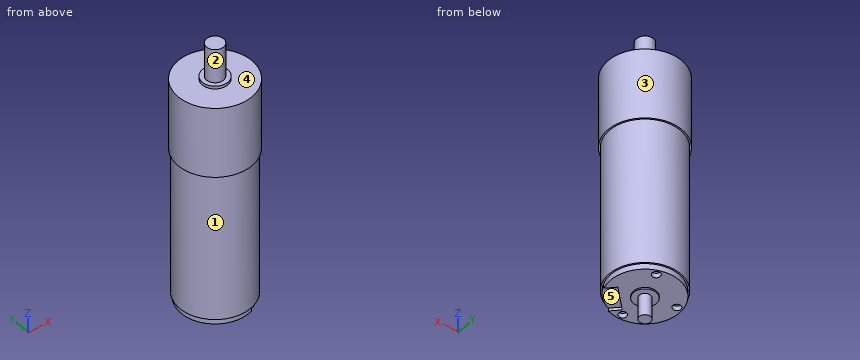
from build123d import *

# Parameters (mm, degrees)
SKETCH3_R          = 2.8
CUT_EXTRUDE2_DEPTH = 3.25
CUT_EXTRUDE3_DEPTH = 2


with BuildPart() as part:
    # Sketch1 → Revolve1 (revolve)
    with BuildSketch(Plane(origin=(0, 0, 0), x_dir=(0, 0, -1), z_dir=(1, 0, 0)), mode=Mode.PRIVATE) as revolve1_sk:
        Polygon((-76, 0), (124.5, 0), (124.5, 4), (109, 4), (109, 8), (108, 8), (108, 24), (104, 24), (104, 25), (0, 25), (0, 26), (-50, 26), (-50, 9), (-52, 9), (-52, 6), (-76, 6), align=None)
    revolve(revolve1_sk.sketch.rotate(Axis((0, 0, 76), (0, 0, -1)), 180), axis=Axis((0, 0, 76), (0, 0, -1)))

    # Sketch3 → Cut-Extrude2 (cut)
    with BuildSketch(Plane.XY.offset(-108)):
        with Locations(Location((6.767859423, 19.032500593, 0), (0, 0, 180))):
            Circle(SKETCH3_R)
        with Locations(Location((-19.905985431, 3.433910891, 0), (0, 0, 180))):
            Circle(SKETCH3_R)
        with Locations(Location((0, -20.2, 0), (0, 0, 180))):
            Circle(SKETCH3_R)
    extrude(amount=CUT_EXTRUDE2_DEPTH, mode=Mode.SUBTRACT)

    # Sketch4 → Cut-Extrude3 (cut)
    with BuildSketch(Plane(origin=(0, 0, -108), x_dir=(-1, 0, 0), z_dir=(0, 0, -1))):
        Polygon((-22.506441861, -8.334271099), (-16.973308635, -2.811902197), (-2.844949371, -16.967800773), (-8.378082597, -22.490169675), (-11.338488517, -25.444816332), (-25.466847781, -11.288917756), align=None)
    extrude(amount=-CUT_EXTRUDE3_DEPTH, mode=Mode.SUBTRACT)


solid = part.part
Could you check a few things on this model? Use its own coordinates, in mm. Face numbers are marked on the shaded views. A direction names the side the tool comes from. Give positions to 0.01 mm unless a question says otherwise; leave off trailing zeros. Loops run counter-clockwise (first coordinate to the right, second up) from the corner with the lowest first, then second, coordinate; pieces in that order, holes last. Notation, with made-up numbers: M -35.5,-1 L -9.5,-1 A12 ccw -9.5,8 Z; hole C -34,-11 d6. An arc over 180 degrees is marked long. Answer as a JSON object with one key per item and string values.
Q1. Suppose I cut it at C-C, the plane y = -20.2. List the corners of the cut face in (x, z) for me.
Values found:
{"outline": "M -16.37,0 L -14.73,0 L -14.73,-104 L -12.96,-104 L -12.96,-108 L -2.8,-108 L -2.8,-104.75 L 2.8,-104.75 L 2.8,-108 L 6.08,-108 L 6.08,-106 L 12.96,-106 L 12.96,-104 L 14.73,-104 L 14.73,0 L 16.37,0 L 16.37,50 L -16.37,50 Z"}
Q2. For P1, Ø15.5, axis at x = 11, y = -13.5, coming from the -Z side; P2, Ø6.5, axis at x = 6.77, y = 19.03, coming from the +Z side; P3, Ø3, axis at y = -14, z = -33.5, coming from the +X side, each with a flat end and sliding along its axis, tell me the tip position at first contact or that it passes through.
Values found:
{"P1": "stops at z = -108", "P2": "stops at z = 50", "P3": "stops at x = 21.65"}
Q3. If we mould it in two halves opening along X, with no side actions, what happens to the marked faces 3, 4 and 5? For each: pulls with the +X half, pulls with the -X half, needs draft (parallel to the pull), parting line crosses it, or undercut.
Values found:
{"face 3": "parting line crosses it", "face 4": "needs draft", "face 5": "undercut"}
Q4. If I drill on probe 1 along Z at (x, y) = (17.5, 15.5); probe 2 along X at (y, z) = (-20.2, -106.15); probe 3 along Z at (x, y) = (4.5, -1), over which ranges is the centre line in solid material (lowest first)? Write a range as [from, to].
Values found:
{"probe 1": "z = [-108, 50]", "probe 2": "x = [-12.96, -2.8], [2.8, 6.08]", "probe 3": "z = [-109, 76]"}
Q5. Suppose I cut it at D-D, the plane z = -90. List the corners of the cut face in (x, y) for me.
Values found:
{"outline": "C 0,0 d50"}
Q6. Suppose I cut it at B-B, the plane z = 7.5. List the corners of the cut face in (x, y) for me, plus the area to 3 significant figures.
Values found:
{"outline": "C 0,0 d52", "area": "2,120 mm²"}
Q7. For the marked faces 1 and 2, which set-ups out of +Z, -Z, +X, -X, +Y, -Y let a thin tool reach every point of the face, with its end or its side?
Values found:
{"face 1": "-Z", "face 2": "+Z"}
